Input: part model. Units: mm. Frame: model coordinates. A direction names the side the tool comes from. Give positions to 0.01 mm unless a question says otherwise; leave off trailing zeros. Loops run counter-clockwise (first coordinate to the right, second up) from the corner with the lowest first, then second, coordinate; pieces in that order, holes last. Notation, with made-up numbers: (-5.5, 27) - (22.5, 27) arc R32 ccw to (22.5, 56) - close; hole circle Ø3 at (65, 20). An arc over 180 degrees is marked (long way). Answer as a JSON object with one key per item and string values.
from build123d import *

# Parameters (mm, degrees)
F0_R     = 707.076711983
F0_R_2   = 575.1975047279
F0_R_3   = 452.5428910843
F1_DEPTH = 203.2
F2_DEPTH = 203.2
F3_SIZE  = 101.6


# Not quite as in the source:
# - a feature names something its author has since deleted; it is built from what else it names


with BuildPart() as f1:
    # F0 (on Top) → F1 (new body)
    with BuildSketch(Plane.XY):
        Circle(F0_R)
        Circle(F0_R_2, mode=Mode.SUBTRACT)
        Circle(F0_R_2)
        Circle(F0_R_3, mode=Mode.SUBTRACT)
        Circle(F0_R_3)
    extrude(amount=-F1_DEPTH)

    # F0 (on Top) → F2 (join)
    with BuildSketch(Plane.XY):
        Circle(F0_R)
        Circle(F0_R_2, mode=Mode.SUBTRACT)
        Circle(F0_R_3)
    extrude(amount=F2_DEPTH)

    # F3
    f3_edges = [f1.edges().sort_by_distance(p)[0] for p in [
        (-707.076712, 0, -203.2),
    ]]
    chamfer(f3_edges, length=F3_SIZE)


solid = f1.part
Item 1: Cut plane B-B (y = 0). Return loops of the section in (x, z), then the cut area to 3 significant figures.
Geometry check:
{"outline": "(-707.08, -101.6) - (-605.48, -203.2) - (605.48, -203.2) - (707.08, -101.6) - (707.08, 203.2) - (575.2, 203.2) - (575.2, 0) - (452.54, 0) - (452.54, 203.2) - (-452.54, 203.2) - (-452.54, 0) - (-575.2, 0) - (-575.2, 203.2) - (-707.08, 203.2) - close", "area": "515,000 mm2"}
Item 2: Material intervals for line 1 (Y direction, x = 0, z = 83); line 2 (X direction, y = -4, z = 185); line 3 (Y direction, x = 365, z = 100), sorted ascending. Write a range as [from, to].
Geometry check:
{"line 1": "y = [-707.08, -575.2], [-452.54, 452.54], [575.2, 707.08]", "line 2": "x = [-707.07, -575.18], [-452.53, 452.53], [575.18, 707.07]", "line 3": "y = [-605.58, -444.55], [-267.53, 267.53], [444.55, 605.58]"}
Item 3: Mould query, pull axis Y, two halves, no side actions, for faces 1 (the face through (431.645, 135.932, 100.178)), 2 (the face through (-6, 6, 203.2)), 3 (the face through (-132.32, -595.89, -198.27)). Classes: released by +Y, released by -Y, zero draft, split by the parting line, or undercut.
Geometry check:
{"face 1": "undercut", "face 2": "zero draft", "face 3": "split by the parting line"}
Item 4: Cut plane A-A (z = 92). Return loops of the section in (x, y) (1 decimal), then the cut area to 3 significant figures.
Geometry check:
{"outline": "circle Ø1414.2 at (0, 0); circle Ø905.1 at (0, 0); hole circle Ø1150.4 at (0, 0)", "area": "1,170,000 mm2"}
Item 5: Access query for faces 4 (the face through (-344, -296, 0)), 5 (the face through (-8, 8, -203.2)). Directions: +Z, -Z, +X, -X, +Y, -Y. A direction counts if a zero-diameter tool reaches every point of the face in a straight line with its end or side. Return the directions, or none.
Geometry check:
{"face 4": "+Z", "face 5": "-Z, +X, -X, +Y, -Y"}
Item 6: Contact query for flat-ended pins moving along their axis: P1, Ø3, axis at x = 449.5, z = -151, coming from the -Y side; P2, Ø8, axis at y = -321, z = -3.5, coming from the -X side; P3, Ø1.5, axis at x = 479.5, y = 508.5, coming from the -Z side. Output: stop coordinate, or through.
Geometry check:
{"P1": "stops at y = -482.58", "P2": "stops at x = -632.04", "P3": "stops at z = -110.5"}
